Can you work these out from the model? Positions are in its coordinate system, mm. A direction names the side the tool comes from. Give positions to 0.01 mm unless a question says otherwise; leave off trailing zeros. Write each loop counter-clockwise with the first axis right and the second up, starting at its lowest first coordinate (ties: lowest second). Pieces come first, ordered by that corner, then holes.
1. I'm going to push flat-ended pins straight in: pin 1 (10 mm diameter, centred on x = -6.5, z = 14, fed in from +Y); pin 2 (5 mm diameter, centred on y = 8, z = -10.5, fed in from -X); pin 3 (0.6 mm diameter, centred on x = -35, z = 21.5, fed in from +Y). Where does each tip first touch, or does it pass through?
2. Thinking about a two-plate mould opening in X: for faces 1 (the flat face through (0, 5, -28)), 2 (the flat face through (0, 7, -27)), 3 (the flat face through (35, 5, 0)), which applies, pulls with the +X half, pulls with the -X half, needs draft (parallel to the pull), parting line crosses it, or undercut?
3. If I drill on probe 1 along Z at (x, y) = (-29, 8.5); probe 2 along X at (y, z) = (5, -9.5); probe 3 along X at (y, z) = (9, -10.5), over which ranges is the centre line in solid material (lowest first)?
4. On a 3-axis mill with a long thin cutter (end or side, diameter ignored), from which of +Z, -Z, +X, -X, +Y, -Y can I reach the whole of each face in a straight line? I mean faces 4 (the flat face through (0, 5, 28)), 5 (the flat face through (0, 7, 27)). Say none if no direction works.
5. Suppose I cut it at A-A (y = 7). Please give me the cut outline in (x, z).
6. Suppose I cut it at C-C (z = -9). Please give me the cut outline in (x, y), and give its area (3 significant figures).
7. Suppose I cut it at B-B (x = -8.5). Please give me the cut outline in (y, z), and give its area (3 significant figures).
```python
from build123d import *

# Parameters (mm, degrees)
SKETCH1_W           = 70
SKETCH1_H           = 56
BOSS_EXTRUDE1_DEPTH = 10
SKETCH2_W           = 69
SKETCH2_H           = 54
CUT_EXTRUDE1_DEPTH  = 6
SKETCH3_W           = 12.993398332
SKETCH3_H           = 10.754862036
SKETCH3_W_2         = 9.953735061
SKETCH3_H_2         = 10.5
CUT_EXTRUDE2_DEPTH  = 10


with BuildPart() as part:
    # Sketch1 → Boss-Extrude1 (new body)
    with BuildSketch(Plane(origin=(0, 0, 0), x_dir=(1, 0, 0), z_dir=(0, 1, 0))):
        Rectangle(SKETCH1_W, SKETCH1_H)
    extrude(amount=BOSS_EXTRUDE1_DEPTH)

    # Sketch2 → Cut-Extrude1 (cut)
    with BuildSketch(Plane(origin=(0, 10, 0), x_dir=(1, 0, 0), z_dir=(0, 1, 0))):
        Rectangle(SKETCH2_W, SKETCH2_H)
    extrude(amount=-CUT_EXTRUDE1_DEPTH, mode=Mode.SUBTRACT)

    # Sketch3 → Cut-Extrude2 (cut)
    with BuildSketch(Plane.ZY.offset(35)):
        with Locations((-11.292948147, 10.977431018)):
            Rectangle(SKETCH3_W, SKETCH3_H)
        with Locations((19.073286927, 10.85)):
            Rectangle(SKETCH3_W_2, SKETCH3_H_2)
    extrude(amount=-CUT_EXTRUDE2_DEPTH, mode=Mode.SUBTRACT)


solid = part.part
```
Checks:
1. pin 1: stops at y = 4
1. pin 2: stops at x = -35
1. pin 3: stops at y = 5.6
2. face 1: needs draft
2. face 2: undercut
2. face 3: pulls with the +X half
3. probe 1: z = -28 to -27, 27 to 28
3. probe 2: x = -35 to -34.5, 34.5 to 35
3. probe 3: x = 34.5 to 35
4. face 4: +Z, +X, -X, +Y, -Y
4. face 5: +Y
5. outline: (-35, -28) - (35, -28) - (35, 28) - (-35, 28) - (-35, 24.05) - (-34.5, 24.05) - (-34.5, 27) - (34.5, 27) - (34.5, -27) - (-34.5, -27) - (-34.5, -17.79) - (-35, -17.79) - close; (-35, -4.8) - (-34.5, -4.8) - (-34.5, 14.1) - (-35, 14.1) - close
6. outline: (-35, 0) - (35, 0) - (35, 10) - (34.5, 10) - (34.5, 4) - (-34.5, 4) - (-34.5, 5.6) - (-35, 5.6) - close
6. area: 284 mm2
7. outline: (0, -28) - (10, -28) - (10, -27) - (4, -27) - (4, 27) - (10, 27) - (10, 28) - (0, 28) - close
7. area: 236 mm2
